Autodesk Inventor part; units mm, degrees
ref_plane "YZ Plane" through (0, 0, 0) normal (1, 0, 0) x (0, 1, 0)
ref_plane "XZ Plane" through (0, 0, 0) normal (0, 1, 0) x (-1, 0, 0)
ref_plane "XY Plane" through (0, 0, 0) normal (0, 0, 1) x (1, 0, 0)
sketch "스케치1" plane through (0, 0, 0) normal (1, 0, 0) x (0, 1, 0)
  line L0 (-15, -8.4) -> (15, -8.4)
  line L1 (15, -8.4) -> (15, -11.4)
  line L2 (15, -11.4) -> (-15, -11.4)
  line L3 (-15, -11.4) -> (-15, -8.4)
  line L4 (-15, -8.4) -> (15, -11.4) construction
  line L5 (15, -8.4) -> (-15, -11.4) construction
  line L6 (-10.7716, 0) -> (20.6854, 0) construction
  circle A0 centre (17.9, 0) radius 5.4
  circle A1 centre (17.9, 0) radius 8.4
  line L7 (9.5, -4.3302) -> (9.5, -23.7251) construction
  line L8 (15, -8.4) -> (17.9, -8.4)
  line L9 (9.5, 0) -> (9.5, -8.4)
  line L10 (56.0253, 38.4) -> (-49.003, 38.4) construction
  line L11 (-15, 85.2) -> (15, 85.2)
  line L12 (15, 85.2) -> (15, 88.2)
  line L13 (15, 88.2) -> (-15, 88.2)
  line L14 (-15, 88.2) -> (-15, 85.2)
  line L15 (-15, 85.2) -> (15, 88.2) construction
  line L16 (15, 85.2) -> (-15, 88.2) construction
  line L17 (-10.7716, 76.8) -> (20.6854, 76.8) construction
  circle A2 centre (17.9, 76.8) radius 5.4
  circle A3 centre (17.9, 76.8) radius 8.4
  line L18 (9.5, 81.1302) -> (9.5, 100.5251) construction
  line L19 (15, 85.2) -> (17.9, 85.2)
  line L20 (9.5, 76.8) -> (9.5, 85.2)
  line L21 (15, -11.4) -> (26.3, -11.4)
  line L22 (26.3, -11.4) -> (26.3, 0)
  line L23 (15, 88.2) -> (26.3, 88.2)
  line L24 (26.3, 88.2) -> (26.3, 76.8)
  point P0 (0, -9.9)
  point P1 (6.5, -8.4)
  point P2 (22.1201, -7.263)
  point P3 (0, 86.7)
  point P4 (6.5, 85.2)
  point P5 (22.1201, 84.063)
  dimension "d2" = 30
  dimension "d3" = 3
  dimension "d9" = 10.8
  dimension "d10" = 16.8
  dimension "d11" = 8.5
  dimension "d12" = 3
  dimension "d20" = 38.4
extrude "돌출1" add sketch "스케치1" along normal mid plane 20
fillet "모깎기1" radius 4 2 edges at (0, 26.3, -11.4) (0, 26.3, 88.2)
sketch "스케치4" plane through (10, -15, -11.4) normal (0, 0, -1) x (-1, 0, 0)
  line L0 (-6.6272, 15) -> (50.9826, 15) construction
  line L1 (10, 54.1091) -> (10, -11.8144) construction
  circle A0 centre (3.5, 8.5) radius 1.5
  line L2 (20, 0) -> (0, 0)
  line L3 (0, 0) -> (0, 37.3)
  circle A1 centre (16.5, 8.5) radius 1.5
  circle A2 centre (3.5, 21.5) radius 1.5
  circle A3 centre (16.5, 21.5) radius 1.5
  circle A4 centre (10, 32.9) radius 1.25
  line L4 (20, 41.3) -> (0, 41.3)
  point P0 (10, 15)
  dimension "d22" = 3
  dimension "d23" = 8.5
  dimension "d24" = 3.5
  dimension "d27" = 2.5
  dimension "d28" = 8.4
extrude "돌출4" cut sketch "스케치4" against normal through all contours A0 | A1 | A2 | A3
sketch "스케치5" plane through (-10, 0, 0) normal (-1, 0, 0) x (0, 0, 1)
  circle A0 centre (0, 17.9) radius 5.4
  arc A1 (-7.4, 26.3) -> (-11.4, 22.3) centre (-7.4, 22.3) ccw
  line L0 (-11.4, 22.3) -> (-11.4, -15)
  line L1 (-11.4, -15) -> (-8.4, -15)
  line L2 (-8.4, -15) -> (-8.4, 9.5)
  line L3 (-8.4, 9.5) -> (0, 9.5)
  arc A2 (0, 9.5) -> (0, 26.3) centre (0, 17.9) ccw
  line L4 (0, 26.3) -> (-7.4, 26.3)
  circle A3 centre (76.8, 17.9) radius 5.4
  arc A4 (88.2, 22.3) -> (84.2, 26.3) centre (84.2, 22.3) ccw
  line L5 (84.2, 26.3) -> (76.8, 26.3)
  arc A5 (76.8, 26.3) -> (76.8, 9.5) centre (76.8, 17.9) ccw
  line L6 (76.8, 9.5) -> (85.2, 9.5)
  line L7 (85.2, 9.5) -> (85.2, -15)
  line L8 (85.2, -15) -> (88.2, -15)
  line L9 (88.2, -15) -> (88.2, 22.3)
  line L10 (-8.4, -15) -> (85.2, -15)
  line L11 (-8.4, -11) -> (85.2, -11)
  line L12 (85.2, -15) -> (88.2, -15)
  line L13 (-8.4, 9.5) -> (-8.4, -15)
  line L14 (0, 26.3) -> (76.8, 26.3)
  circle A6 centre (0, 17.9) radius 5.4
  circle A7 centre (76.8, 17.9) radius 5.4
  line L15 (-8.4, -2.062) -> (85.2, -2.062) construction
  line L16 (-8.4, -4.062) -> (85.2, -4.062)
  line L17 (7.1554, 22.3) -> (69.6446, 22.3)
  line L18 (-8.4, -0.062) -> (85.2, -0.062)
  point P0 (0, 0)
  point P1 (0, -6.5)
  point P2 (0, 6.5)
  point P3 (0, 0)
  dimension "d29" = 4
  dimension "d31" = 8.5
  dimension "d32" = 13
  dimension "d33" = 6.5
  dimension "d34" = 2
  dimension "d35" = 4
extrude "돌출5" add sketch "스케치5" against normal up to surface (20 mm away) contours L14 A5 L17 A2 | L2 L11 L7 L10 | L2 L18 L7 L16
sketch "스케치6" plane through (-10, -15, -11.4) normal (0, -1, 0) x (1, 0, 0)
  circle A0 centre (10, 10) radius 5
  line L0 (0, 0) -> (20, 0)
  line L1 (10, 10) -> (10, 54.4458) construction
  circle A1 centre (10, 89.6) radius 5
  line L2 (0, 99.6) -> (20, 99.6)
  circle A2 centre (10, 30) radius 5
  circle A3 centre (10, 69.6) radius 5
  circle A4 centre (10, 49.6) radius 5
  point P0 (10, 11.4)
  dimension "d38" = 10
  dimension "d39" = 10
  dimension "d40" = 10
  dimension "d41" = 10
  dimension "d44" = 20
  dimension "d51" = 20
extrude "돌출6" cut sketch "스케치6" against normal up to surface (14.938 mm away)
extrude "돌출7" cut sketch "스케치6" against normal through all contours A2 | A3 | A4
sketch "스케치7" plane through (-10, 0, 0) normal (-1, 0, 0) x (0, 0, 1)
  arc A0 (0, 9.5) -> (7.1554, 22.3) centre (0, 17.9) ccw
  arc A1 (69.6446, 22.3) -> (76.8, 9.5) centre (76.8, 17.9) ccw
  line L0 (-8.4, 9.5) -> (0, 9.5)
  line L1 (-11.4, 22.3) -> (-11.4, -15)
  arc A2 (-7.4, 26.3) -> (-11.4, 22.3) centre (-7.4, 22.3) ccw
  line L2 (84.2, 26.3) -> (-7.4, 26.3)
  arc A3 (88.2, 22.3) -> (84.2, 26.3) centre (84.2, 22.3) ccw
  line L3 (88.2, -15) -> (88.2, 22.3)
  line L4 (76.8, 9.5) -> (85.2, 9.5)
  line L5 (-8.4, 9.5) -> (-11.4, 9.5)
  line L6 (85.2, 9.5) -> (88.2, 9.5)
  arc A4 (7.1554, 22.3) -> (0, 26.3) centre (0, 17.9) ccw
  line L7 (7.1554, 22.3) -> (69.6446, 22.3)
  arc A5 (76.8, 26.3) -> (69.6446, 22.3) centre (76.8, 17.9) ccw
  circle A6 centre (0, 17.9) radius 5.4
  circle A7 centre (76.8, 17.9) radius 5.4
  point P0 (0, 0)
extrude "돌출8" add sketch "스케치7" along normal blind 10 contours L0 L5 L1 A2 L2 A4 A0 | A5 L2 A3 L3 L6 L4 A1
sketch "스케치8" plane through (10, 0, 0) normal (1, 0, 0) x (0, 0, -1)
  line L0 (0, 9.5) -> (8.4, 9.5)
  arc A0 (-7.1554, 22.3) -> (0, 9.5) centre (0, 17.9) ccw
  arc A1 (0, 26.3) -> (-7.1554, 22.3) centre (0, 17.9) ccw
  line L1 (7.4, 26.3) -> (-84.2, 26.3)
  arc A2 (11.4, 22.3) -> (7.4, 26.3) centre (7.4, 22.3) ccw
  line L2 (11.4, -15) -> (11.4, 22.3)
  circle A3 centre (0, 17.9) radius 5.4
  line L3 (8.4, 9.5) -> (11.4, 9.5)
  arc A4 (-76.8, 9.5) -> (-69.6446, 22.3) centre (-76.8, 17.9) ccw
  line L4 (-85.2, 9.5) -> (-76.8, 9.5)
  arc A5 (-69.6446, 22.3) -> (-76.8, 26.3) centre (-76.8, 17.9) ccw
  arc A6 (-84.2, 26.3) -> (-88.2, 22.3) centre (-84.2, 22.3) ccw
  circle A7 centre (-76.8, 17.9) radius 5.4
  line L5 (-88.2, 9.5) -> (-85.2, 9.5)
  line L6 (-88.2, 22.3) -> (-88.2, -15)
  point P0 (0, 0)
extrude "돌출9" add sketch "스케치8" along normal blind 10
sketch "스케치9" plane through (10, -15, -11.4) normal (0, 0, -1) x (-1, 0, 0)
  circle A0 centre (16.5, 8.5) radius 1.5
  circle A1 centre (3.5, 8.5) radius 1.5
  circle A2 centre (3.5, 21.5) radius 1.5
  circle A3 centre (16.5, 21.5) radius 1.5
  line L0 (-10, 37.3) -> (30, 37.3)
  line L1 (-10, 24.5) -> (-10, 37.3)
  line L2 (0, 24.5) -> (-10, 24.5)
  line L3 (0, 0) -> (0, 24.5)
  line L4 (20, 0) -> (0, 0)
  line L5 (20, 24.5) -> (20, 0)
  line L6 (20, 24.5) -> (30, 24.5)
  line L7 (30, 37.3) -> (30, 24.5)
  line L8 (5, 37.3) -> (5, 41.3)
  line L9 (5, 37.3) -> (5, 41.3)
  line L10 (5, 37.3) -> (5, 41.3)
  line L11 (30, 41.3) -> (-10, 41.3)
  line L12 (-10, 37.3) -> (30, 37.3)
  line L13 (30, 41.3) -> (30, 37.3)
  line L14 (30, 41.3) -> (-10, 41.3)
  line L15 (-10, 37.3) -> (-10, 41.3)
  line L16 (-10, 32.9) -> (30, 32.9) construction
  circle A4 centre (-5, 32.9) radius 1.25
  circle A5 centre (25, 32.9) radius 1.25
  point P0 (10, 15)
  dimension "d64" = 8.4
  dimension "d65" = 2.5
  dimension "d66" = 2.5
  dimension "d67" = 5
  dimension "d68" = 5
properties part number "top"
Model file for the job. Use its own axes, mm. A direction names the side the tool comes from. Coordinates: 2 decimals unless noted, no trailing zeros. Write each loop counter-clockwise with the first axis right and the second up, starting at its lowest first coordinate (ties: lowest second). Pieces come first, ordered by that corner, then holes. Notation, with made-up numbers: (-21, 6.25) - (-7, 6.25) arc R20 ccw to (-7, 22.25) - close; hole circle Ø5 at (13.25, -24). An arc over 180 degrees is marked (long way). One line per item, written item: value. Start each with the question number.
1. Flat gauge pins, fed straight in: pin 1 (5 mm diameter, centred on y = 19, z = 67, fed in from +X); pin 2 (3 mm diameter, centred on y = -2, z = 34.5, fed in from -X); pin 3 (3 mm diameter, centred on y = 25, z = 35, fed in from +X). Where does each tip first touch, or does it go through?
2. Slice it at C-C (z = 12.5). Write the cut outline in (x, y).
3. Slice it at D-D (y = 2.5). Write the cut outline in (x, z).
4. Slice it at A-A (x = -17.5). Write the cut outline in (y, z), plus the area to 3 significant figures.
5. Probe line 1 (Y direction, x = 3.5, z = 28.5); line 2 (X direction, y = -2, z = 38); line 3 (Z direction, x = -9, y = 4.5). List the from-to ranges inside material, lowest first. Write a range as from..to.
6. Slice it at B-B (y = -6.5). Write the cut outline in (x, z), plus the area to 3 significant figures.
7. Mould opens along Z. For faces 1 (the cylindrical face through (-5.3, 5.6, 86.7)), 2 (the cylindrical face through (-0.651, -13.028, 23.557)), 3 (the flat face through (0, 8, 88.2)), 4 (the cylindrical face through (-1.08, -13.03, 53.32)) say: released by +Z, released by -Z, zero draft, split by the parting line, or undercut.
8. Tool access for faces 5 (the cylindrical face through (-5.3, -7.4, 86.7)), 6 (the cylindrical face through (-1.08, 24.27, 53.32)), 7 (the cylindrical face through (-1.08, -2.09, 73.32)), 8 (the flat face through (-7, -11, 38)), 9 (the flat face through (-10, -3, 39)): list every direction of +Z, -Z, +X, -X, +Y, -Y with a clear straight run to the whole face (end or side of a thin tool).
Answers below:
1. pin 1: stops at x = 20
1. pin 2: stops at x = -10
1. pin 3: stops at x = 10
2. outline: (-10, -15) - (10, -15) - (10, -11) - (-10, -11) - close; (-10, -4.06) - (10, -4.06) - (10, -0.06) - (-10, -0.06) - close; (-10, 22.3) - (10, 22.3) - (10, 26.3) - (-10, 26.3) - close
3. outline: (-10, -11.4) - (10, -11.4) - (10, -8.4) - (-10, -8.4) - close; (-10, 85.2) - (10, 85.2) - (10, 88.2) - (-10, 88.2) - close
4. outline: (9.5, -11.4) - (22.3, -11.4) arc R4 ccw to (26.3, -7.4) - (26.3, 0) arc R8.4 ccw to (22.3, 7.16) arc R8.4 ccw to (9.5, 0) - close; (9.5, 76.8) arc R8.4 ccw to (22.3, 69.64) arc R8.4 ccw to (26.3, 76.8) - (26.3, 84.2) arc R4 ccw to (22.3, 88.2) - (9.5, 88.2) - close; hole circle Ø10.8 at (17.9, 0); hole circle Ø10.8 at (17.9, 76.8)
4. area: 415 mm^2
5. line 1: y = -15..-11, -4.06..-0.06, 22.3..26.3
5. line 2: x = -10..-5, 5..10
5. line 3: z = -11.4..-8.4, 85.2..88.2
6. outline: (-10, -11.4) - (-8, -11.4) - (-8, -8.4) - (-10, -8.4) - close; (-10, 85.2) - (-8, 85.2) - (-8, 88.2) - (-10, 88.2) - close; (-5, -11.4) - (5, -11.4) - (5, -8.4) - (-5, -8.4) - close; (-5, 85.2) - (5, 85.2) - (5, 88.2) - (-5, 88.2) - close; (8, -11.4) - (10, -11.4) - (10, -8.4) - (8, -8.4) - close; (8, 85.2) - (10, 85.2) - (10, 88.2) - (8, 88.2) - close
6. area: 84.0 mm^2
7. face 1: zero draft
7. face 2: undercut
7. face 3: released by +Z
7. face 4: undercut
8. face 5: +Z, -Z
8. face 6: +Y, -Y
8. face 7: -Y
8. face 8: +X, -X
8. face 9: +Z, -Z, -X, -Y
